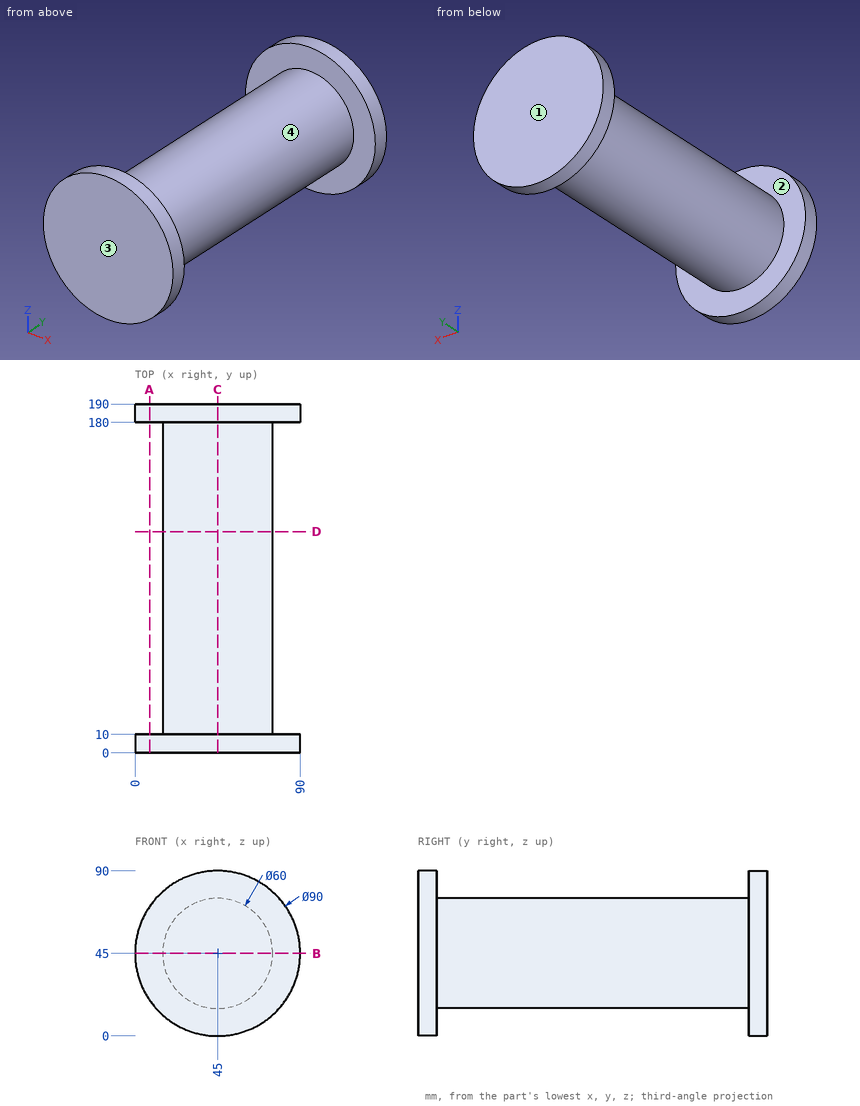
Source: three-view drawing plus pictorial views. Frame: mm from the lowest corner of the part. Coordinates: 2 decimals unless noted, no trailing zeros. Order: outer loops, then holes, each group sorted by start corner. A loop starts at its lowest first (then second) coordinate and runs counter-clockwise, first axis right, second up. Notation, with made-up numbers: M 3,-16.5 L 32,-16.5 A9 ccw 32,-12.5 Z; hole C 74.25,14.25 d1. An arc over 180 degrees is marked long. One line per question, with ' | ' between items.
Item 1: Pin query (flat end, axial travel): pin 1 (8 mm diameter, centred on y = 76.5, z = 48, fed in from +X); pin 2 (3 mm diameter, centred on x = 64.5, y = 44.5, fed in from +Z); pin 3 (6 mm diameter, centred on x = 20.5, y = 43, fed in from -Z). Return the tip coordinate at first contact, or that it passes through.
Geometry results:
pin 1: stops at x = 75 | pin 2: stops at z = 69 | pin 3: stops at z = 24.08
Item 2: Draft query along Y for the marked faces 1, 2, 3 and 4. Return one class per face: released by +Y, released by -Y, zero draft, split by the parting line, or undercut.
Geometry results:
face 1: released by +Y | face 2: undercut | face 3: released by -Y | face 4: undercut
Item 3: Section B-B (z = 45). Output: boundary loops of the cut face in (x, y), then the cut area to 3 significant figures.
Geometry results:
outline: M 0,0 L 90,0 L 90,10 L 75,10 L 75,180 L 90,180 L 90,190 L 0,190 L 0,180 L 15,180 L 15,10 L 0,10 Z | area: 12,000 mm^2
Item 4: Section A-A (x = 8). Output: boundary loops of the cut face in (y, z), then the cut area to 3 significant figures.
Geometry results:
outline: M 0,19.39 L 10,19.39 L 10,70.61 L 0,70.61 Z; M 180,19.39 L 190,19.39 L 190,70.61 L 180,70.61 Z | area: 1,020 mm^2
Item 5: Ray query, line 1 along Y through (x, z) = (58.5, 17); line 2 along Z through (x, y) = (46, 69.5); line 3 along X through (y, z) = (88, 39.5). Return the intervals inside material, ascending.
Geometry results:
line 1: y = 0 to 10, 180 to 190 | line 2: z = 15.02 to 74.98 | line 3: x = 15.51 to 74.49
Item 6: Section D-D (y = 120.5). Output: boundary loops of the cut face in (x, z).
Geometry results:
outline: C 45,45 d60
Item 7: Section C-C (x = 45). Output: boundary loops of the cut face in (y, z), then the cut area to 3 significant figures.
Geometry results:
outline: M 0,0 L 10,0 L 10,15 L 180,15 L 180,0 L 190,0 L 190,90 L 180,90 L 180,75 L 10,75 L 10,90 L 0,90 Z | area: 12,000 mm^2
